```python
from build123d import *

# Parameters (mm, degrees)
HOLE_WIZARD_M5_1_D  = 4.2
SKETCH_6_W          = 0.6
SKETCH_6_H          = 4.214261502
CUT_EXTRUDE_1_DEPTH = 4


with BuildPart() as part:
    # 草图1 → 旋转1 (revolve)
    with BuildSketch(Plane(origin=(0, 0, 0), x_dir=(1, 0, 0), z_dir=(0, 1, 0)), mode=Mode.PRIVATE) as revolve_1_sk:
        Polygon((0, 0), (0, 6), (2.5, 6), (2.5, 3), (5.5, 3), (5.5, 6), (8, 6), (8, 4), (12, 4), (12, 0), align=None)
    revolve(revolve_1_sk.sketch.rotate(Axis((-1000, 0, 0), (1, 0, 0)), 180), axis=Axis((-1000, 0, 0), (1, 0, 0)))

    # M5 螺纹孔1 (through all)
    with Locations(Plane(origin=(12, 0, 0), x_dir=(0, 0, -1), z_dir=(1, 0, 0))):
        with Locations((0, 0)):
            Hole(HOLE_WIZARD_M5_1_D / 2)

    # 草图6 → 切除-拉伸1 (cut)
    with BuildSketch(Plane(origin=(12, 0, 0), x_dir=(0, 0, -1), z_dir=(1, 0, 0))):
        with Locations((-3.7, 0)):
            Rectangle(SKETCH_6_W, SKETCH_6_H)
        with Locations((3.7, 0)):
            Rectangle(SKETCH_6_W, SKETCH_6_H)
    extrude(amount=-CUT_EXTRUDE_1_DEPTH, mode=Mode.SUBTRACT)


solid = part.part
```
Can you work these out from the model? Positions are in its coordinate system, mm. A direction names the side the tool comes from. Round coordinates to 2 decimals unless told otherwise and drop trailing zeros. Order: outer loops, then holes, each group sorted by start corner. A loop starts at its lowest first (then second) coordinate and runs counter-clockwise, first axis right, second up.
(1) If we section it at C-C (x = 10.75): Please give me the cut outline in (y, z).
Results are:
outline: (-2.11, -3.4) - (2.11, -3.4) arc R4 ccw to (2.11, 3.4) - (-2.11, 3.4) arc R4 ccw to start; hole circle Ø4.2 at (0, 0)
(2) If we section it at A-A (z = 0): Please give me the cut outline in (x, y).
Results are:
outline: (0, -6) - (2.5, -6) - (2.5, -3) - (5.5, -3) - (5.5, -6) - (8, -6) - (8, -4) - (12, -4) - (12, -2.1) - (0, -2.1) - close; (0, 2.1) - (12, 2.1) - (12, 4) - (8, 4) - (8, 6) - (5.5, 6) - (5.5, 3) - (2.5, 3) - (2.5, 6) - (0, 6) - close
(3) If we section it at B-B (y = 0): Please give me the cut outline in (x, z).
Results are:
outline: (0, -6) - (2.5, -6) - (2.5, -3) - (5.5, -3) - (5.5, -6) - (8, -6) - (8, -3.4) - (12, -3.4) - (12, -2.1) - (0, -2.1) - close; (0, 2.1) - (12, 2.1) - (12, 3.4) - (8, 3.4) - (8, 6) - (5.5, 6) - (5.5, 3) - (2.5, 3) - (2.5, 6) - (0, 6) - close
(4) If we section it at D-D (z = 2.5): Please give me the cut outline in (x, y), plus the area to 3 significant figures.
Results are:
outline: (0, -5.45) - (2.5, -5.45) - (2.5, -1.66) - (5.5, -1.66) - (5.5, -5.45) - (8, -5.45) - (8, -3.12) - (12, -3.12) - (12, 3.12) - (8, 3.12) - (8, 5.45) - (5.5, 5.45) - (5.5, 1.66) - (2.5, 1.66) - (2.5, 5.45) - (0, 5.45) - close
area: 89.5 mm2
(5) On a 3-axis mill with a long thin cutter (end or side, diameter ignored), from which of +Z, -Z, +X, -X, +Y, -Y can I reach the whole of each face in a straight line? I mean faces 1 (the face through (10, 0, -3.4)), 2 (the face through (10, 0, 3.4)), 3 (the face through (8, 0, -4)), 4 (the face through (10, -4, 0)), 5 (the face through (2.5, 1, -3)). Say none if no direction works.
Results are:
face 1: -Z, +X, +Y, -Y
face 2: +Z, +X, +Y, -Y
face 3: +X
face 4: +X, -Y
face 5: none
(6) If I drill on L1, parallel to X at y = -4.5, z = 0.25; L2, parallel to Y at x = 4.25, z = 0; L3, parallel to X at y = -3.75, z = 0.25, over which ranges is the centre line in solid material (lowest first)?
Results are:
L1: x = 0 to 2.5, 5.5 to 8
L2: y = -3 to -2.1, 2.1 to 3
L3: x = 0 to 2.5, 5.5 to 12
(7) I'm going to push flat-ended pins straight in: pin 1 (1.2 mm diameter, centred on x = 10, y = -0.5, fed in from +Z); pin 2 (3 mm diameter, centred on x = 8.5, y = 2, fed in from -Z); pin 3 (2 mm diameter, centred on x = 10, z = 1.5, fed in from -Y). Where does each tip first touch, or does it pass through?
Results are:
pin 1: stops at z = 3.4
pin 2: stops at z = -5.97
pin 3: stops at y = -3.97
(8) We'd pull the mould along Y, two halves only. Please class faces 6 (the face through (5.5, -3, -1)), 7 (the face through (5.916, 0.631, 2.003)), 8 (the face through (10, 4, 0)): +Y half, -Y half, draft (parallel to the pull), parting line (faces both ways), or undercut.
Results are:
face 6: draft
face 7: undercut
face 8: +Y half
